For this review, take the finished solid that the model builds, in its own axes (mm). A direction names the side the tool comes from. Round coordinates to 2 decimals unless told otherwise and drop trailing zeros. Order: outer loops, then holes, each group sorted by start corner. A loop starts at its lowest first (then second) coordinate and runs counter-clockwise, first axis right, second up. Notation, with made-up numbers: (-36, 43) -> (-30, 43) arc R11 cw to (-30, 58) -> close; hole circle Ø1 at (-36, 44). An arc over 180 degrees is marked (long way). Use a Markdown table: item, result. Add a question column.
1) Consider section C-C (z = -51.5). State the section outline as (x, y) points, plus the area to 3 significant figures.
2) Consider section B-B (y = -7). Give the number of separate pieces and of enclosed holes in the cut face, plus the area to 3 significant figures.
3) Consider section A-A (x = 0). State the section outline as (y, z) points.
4) Draft analysis for pull direction Z (two halves, no side actions). For faces 1 (the face through (13, -12.7, 1)), 2 (the face through (-13.77, -6.26, -61.99)), 3 (the face through (-11.66, -6.26, -3.7)), state which applies: pulls with the +Z half, pulls with the -Z half, needs draft (parallel to the pull), parting line crosses it, or undercut.
5) Clearance check with flat-ended pins moving along their axes: P1, Ø6, axis at y = -6.5, z = 11.5, coming from the +X side; P2, Ø3, axis at x = 3.5, y = -2.5, coming from the +Z side. State where each tip first meets the part, or that it passes through.
6) Machinability: for faces 4 (the face through (-32.09, -6.261, 15.234)), 5 (the face through (13, 0, 1)), which of the approach directions +Z, -Z, +X, -X, +Y, -Y give a long, thin tool a straight path to every point of the face, cutting with its end or side? Answer none if there is none.
7) Consider section D-D (z = 41.5). State the section outline as (x, y) points, plus the area to 3 significant figures.
8) Wall thickness on line 1 along Z through (x, y) = (0, -9); line 2 along X through (y, z) = (-2.75, 23); line 3 along Z through (x, y) = (-2, -3.75): over which ranges is each line inside the solid? List them lowest first. Write a range as [from, to].
```python
from build123d import *

# Parameters (mm, degrees)
F0_R     = 63.5
F0_R_2   = 7.9375
F1_DEPTH = 12.7


with BuildPart() as f1:
    # F0 (on Front) → F1 (new body)
    with BuildSketch(Plane.XZ):
        Circle(F0_R)
        with BuildLine():
            ThreePointArc((54.6665564179, 12.9575831816), (55.8012817771, 6.5229061418), (56.1812366587, 0))
            ThreePointArc((56.1812366587, 0), (51.0550069931, -23.4460575244), (36.6117986709, -42.613466775))
            ThreePointArc((36.6117986709, -42.613466775), (33.0225023635, -45.4515752219), (29.2141472743, -47.988175122))
            ThreePointArc((29.2141472743, -47.988175122), (0, -56.1812366587), (-29.2141472743, -47.988175122))
            ThreePointArc((-29.2141472743, -47.988175122), (-33.0225023635, -45.4515752219), (-36.6117986709, -42.613466775))
            ThreePointArc((-36.6117986709, -42.613466775), (-53.4315312178, -17.3609568925), (-54.6671346388, 12.9551434915))
            ThreePointArc((-54.6671346388, 12.9551434915), (-53.4315312178, 17.3609568925), (-51.8414832422, 21.6516042765))
            ThreePointArc((-51.8414832422, 21.6516042765), (-33.0225023635, 45.4515752219), (-4.572, 55.9948941289))
            ThreePointArc((-4.572, 55.9948941289), (0, 56.1812366587), (4.572, 55.9948941289))
            ThreePointArc((4.572, 55.9948941289), (33.0214881574, 45.4523120685), (51.8405169309, 21.6539178173))
            ThreePointArc((51.8405169309, 21.6539178173), (53.4307563802, 17.3633414164), (54.6665564179, 12.9575831816))
        make_face(mode=Mode.SUBTRACT)
        with BuildLine():
            Line((15.7095408853, 0.2970539508), (54.6665564179, 12.9575831816))
            ThreePointArc((54.6665564179, 12.9575831816), (53.4307563802, 17.3633414164), (51.8405169309, 21.6539178173))
            Line((51.8405169309, 21.6539178173), (12.8846263398, 8.993754178))
            ThreePointArc((12.8846263398, 8.993754178), (7.189720352, 9.8954715726), (4.572, 15.0328433354))
            Line((4.572, 15.0328433354), (4.572, 55.9948941289))
            ThreePointArc((4.572, 55.9948941289), (0, 56.1812366587), (-4.572, 55.9948941289))
            Line((-4.572, 55.9948941289), (-4.572, 15.0328433354))
            ThreePointArc((-4.572, 15.0328433354), (-7.1895636479, 9.8955854211), (-12.8842579143, 8.9936344569))
            Line((-12.8842579143, 8.9936344569), (-51.8414832422, 21.6516042765))
            ThreePointArc((-51.8414832422, 21.6516042765), (-53.4315312178, 17.3609568925), (-54.6671346388, 12.9551434915))
            Line((-54.6671346388, 12.9551434915), (-15.7099093108, 0.2971736719))
            ThreePointArc((-15.7099093108, 0.2971736719), (-11.6329583467, -3.7797772923), (-12.5349093108, -9.4744715586))
            Line((-12.5349093108, -9.4744715586), (-36.6117986709, -42.613466775))
            ThreePointArc((-36.6117986709, -42.613466775), (-33.0225023635, -45.4515752219), (-29.2141472743, -47.988175122))
            Line((-29.2141472743, -47.988175122), (-15.8198157406, -29.5524593622))
            Line((-15.8198157406, -29.5524593622), (-5.1372579143, -14.8491799056))
            ThreePointArc((-5.1372579143, -14.8491799056), (0, -12.2316162576), (5.1372579143, -14.8491799056))
            Line((5.1372579143, -14.8491799056), (29.2141472743, -47.988175122))
            ThreePointArc((29.2141472743, -47.988175122), (33.0225023635, -45.4515752219), (36.6117986709, -42.613466775))
            Line((36.6117986709, -42.613466775), (12.5349093108, -9.4744715586))
            ThreePointArc((12.5349093108, -9.4744715586), (11.6328984945, -3.7799615078), (15.7095408853, 0.2970539508))
        make_face()
        Circle(F0_R_2, mode=Mode.SUBTRACT)
    extrude(amount=F1_DEPTH)


solid = f1.part
```
Results list:
| question | item | result |
|---|---|---|
| 1 | outline | (-37.15, -12.7) -> (-22.45, -12.7) -> (-22.45, 0) -> (-37.15, 0) -> close; (22.45, -12.7) -> (37.15, -12.7) -> (37.15, 0) -> (22.45, 0) -> close |
| 1 | area | 373 mm2 |
| 2 | separate pieces | 1 |
| 2 | enclosed holes | 6 |
| 2 | area | 5,060 mm2 |
| 3 | outline | (-12.7, -63.5) -> (0, -63.5) -> (0, -56.18) -> (-12.7, -56.18) -> close; (-12.7, -12.23) -> (0, -12.23) -> (0, -7.94) -> (-12.7, -7.94) -> close; (-12.7, 7.94) -> (0, 7.94) -> (0, 63.5) -> (-12.7, 63.5) -> close |
| 4 | face 1 | needs draft |
| 4 | face 2 | parting line crosses it |
| 4 | face 3 | undercut |
| 5 | P1 | x = 62.93 |
| 5 | P2 | z = 63.47 |
| 6 | face 4 | +Y, -Y |
| 6 | face 5 | +Z, -Z, +X, -X, +Y |
| 7 | outline | (-48.06, -12.7) -> (-37.87, -12.7) -> (-37.87, 0) -> (-48.06, 0) -> close; (-4.57, -12.7) -> (4.57, -12.7) -> (4.57, 0) -> (-4.57, 0) -> close; (37.87, -12.7) -> (48.06, -12.7) -> (48.06, 0) -> (37.87, 0) -> close |
| 7 | area | 375 mm2 |
| 8 | line 1 | [-63.5, -56.18], [-12.23, -7.94], [7.94, 63.5] |
| 8 | line 2 | [-59.19, -51.26], [-4.57, 4.57], [51.26, 59.19] |
| 8 | line 3 | [-63.47, -56.15], [-12.55, -7.68], [7.68, 63.47] |
